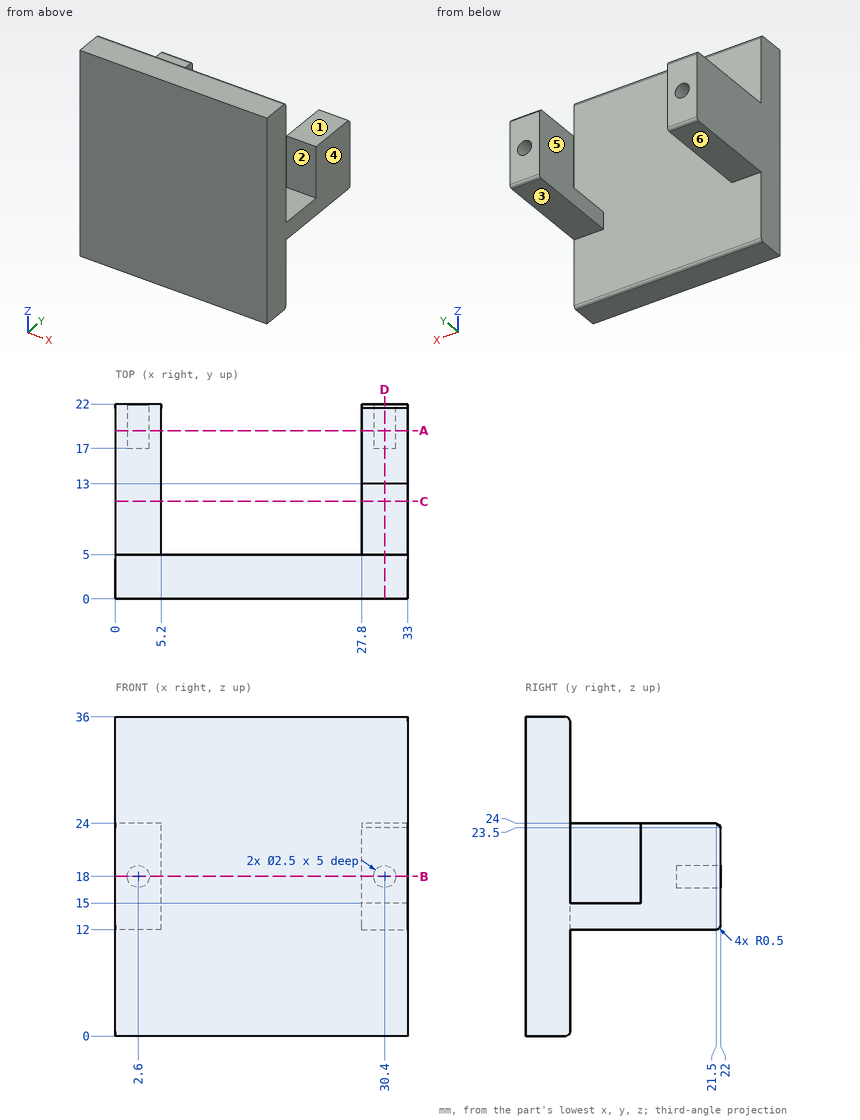
Geometry: see drawing. Coordinates: mm, zero at the bounding-box minimum. A direction names the side the tool comes from. Give positions to 0.01 mm unless a question says otherwise; leave off trailing zeros. Loops run counter-clockwise (first coordinate to the right, second up) from the corner with the lowest first, then second, coordinate; pieces in that order, holes last. Notation, with made-up numbers: (-10, 78.5) - (35, 78.5) arc R29 cw to (35, 108.5) - close; hole circle Ø9 at (-8, 39.25). An arc over 180 degrees is marked (long way). One line per question, with ' | ' between items. Start each with the question number.
(1) Pull-direction query (X, two-part tool) for the marked faces 4, 5 and 6; classes: released by +X, released by -X, zero draft, split by the parting line, or undercut.
(2) Reachability of the marked faces 1, 2 and 3 from +Z, -Z, +X, -X, +Y, -Y: full face, straight path, thin tool, end or side. Return the list, or none.
(3) Ray query, line 1 (Y direction, x = 28, z = 21); line 2 (Z direction, x = 2.6, y = 20.2); line 3 (X direction, y = 8.75, z = 14.5). Return the intervals inside material, ascending. Write a range as from..to.
(4) Contact query for flat-ended pins moving along their axis: pin 1 (5.5 mm diameter, centred on x = 31, y = 16.5, fed in from +Z); pin 2 (4 mm diameter, centred on x = 1.5, y = 14, fed in from -Z); pin 3 (5.5 mm diameter, centred on x = 30, y = 8.5, fed in from +Z). Output: stop coordinate, or through.
(5) Section query A-A on y = 19. Return loops of the section in (x, z).
(6) Section query C-C on y = 11. Return loops of the section in (x, z).
(7) Section query D-D on x = 30.4. Return loops of the section in (y, z), then the cut area to 3 significant figures.
(8) Section query B-B on z = 18. Return loops of the section in (x, y), then the cut area to 3 significant figures.
The answers:
1) face 4: released by +X | face 5: undercut | face 6: zero draft
2) face 1: +Z, +X, -X, +Y | face 2: +Z, +X | face 3: -Z, +X, -X, +Y
3) line 1: 0..5, 13..22 | line 2: 12..16.75, 19.25..24 | line 3: 0..5.2, 27.8..33
4) pin 1: z = 24 | pin 2: z = 12 | pin 3: z = 15
5) outline: (0, 12) - (5.2, 12) - (5.2, 24) - (0, 24) - close; (27.8, 12) - (33, 12) - (33, 24) - (27.8, 24) - close; hole circle Ø2.5 at (2.6, 18); hole circle Ø2.5 at (30.4, 18)
6) outline: (0, 12) - (5.2, 12) - (5.2, 24) - (0, 24) - close; (27.8, 12) - (33, 12) - (33, 15) - (27.8, 15) - close
7) outline: (0, 0) - (4.5, 0) arc R0.5 ccw to (5, 0.5) - (5, 12) - (21.5, 12) arc R0.5 ccw to (22, 12.5) - (22, 16.75) - (17, 16.75) - (17, 19.25) - (22, 19.25) - (22, 23.5) - (21.5, 24) - (13, 24) - (13, 15) - (5, 15) - (5, 35.5) arc R0.5 ccw to (4.5, 36) - (0, 36) - close | area: 299 mm2
8) outline: (0, 0) - (33, 0) - (33, 5) - (5.2, 5) - (5.2, 22) - (3.85, 22) - (3.85, 17) - (1.35, 17) - (1.35, 22) - (0, 22) - close; (27.8, 13) - (33, 13) - (33, 22) - (31.65, 22) - (31.65, 17) - (29.15, 17) - (29.15, 22) - (27.8, 22) - close | area: 275 mm2
